```python
from build123d import *

# Parameters (mm, degrees)
SZKIC2_W                    = 62
SZKIC2_H                    = 5
SZKIC3_R                    = 1.45
DODANIE_WYCI_GNI_CIE1_DEPTH = 5
SFAZOWANIE1_SIZE            = 4
ZAOKR_GLENIE1_R             = 2
SFAZOWANIE2_SIZE            = 0.5


with BuildPart() as part:
    # Szkic2 → Obrót1 (revolve)
    with BuildSketch(Plane.XY):
        Polygon((15, 15), (15, 5), (25, 5), (25, 25), (8.15, 25), (8.15, 15), align=None)
        with Locations((46, 2.5)):
            Rectangle(SZKIC2_W, SZKIC2_H)
    revolve(axis=Axis((0, 0, 0), (0, 1, 0)))

    # Szkic3 → Dodanie-wyciągnięcie1 (add)
    with BuildSketch(Plane(origin=(0, 5, 0), x_dir=(1, 0, 0), z_dir=(0, 1, 0))):
        with BuildLine():
            Line((-4, 76.5), (-4, 79))
            ThreePointArc((-4, 79), (0, 83), (4, 79))
            Line((4, 79), (4, 76.5))
            ThreePointArc((4, 76.5), (0, 72.5), (-4, 76.5))
        make_face()
        with Locations((0, 79)):
            Circle(SZKIC3_R, mode=Mode.SUBTRACT)
        with BuildLine():
            Line((76.5, 4), (79, 4))
            ThreePointArc((79, 4), (83, 0), (79, -4))
            Line((79, -4), (76.5, -4))
            ThreePointArc((76.5, -4), (72.5, 0), (76.5, 4))
        make_face()
        with Locations((79, 0)):
            Circle(SZKIC3_R, mode=Mode.SUBTRACT)
        with BuildLine():
            Line((4, -76.5), (4, -79))
            ThreePointArc((4, -79), (0, -83), (-4, -79))
            Line((-4, -79), (-4, -76.5))
            ThreePointArc((-4, -76.5), (0, -72.5), (4, -76.5))
        make_face()
        with Locations((0, -79)):
            Circle(SZKIC3_R, mode=Mode.SUBTRACT)
        with BuildLine():
            Line((-76.5, -4), (-79, -4))
            ThreePointArc((-79, -4), (-83, 0), (-79, 4))
            Line((-79, 4), (-76.5, 4))
            ThreePointArc((-76.5, 4), (-72.5, 0), (-76.5, -4))
        make_face()
        with Locations((-79, 0)):
            Circle(SZKIC3_R, mode=Mode.SUBTRACT)
    extrude(amount=-DODANIE_WYCI_GNI_CIE1_DEPTH)

    # Sfazowanie1
    sfazowanie1_edges = [part.edges().sort_by_distance(p)[0] for p in [
        (-25, 25, 0),
        (-25, 5, 0),
    ]]
    chamfer(sfazowanie1_edges, length=SFAZOWANIE1_SIZE)

    # Zaokrąglenie1
    zaokr_glenie1_edges = [part.edges().sort_by_distance(p)[0] for p in [
        (-76.896033708, 2.5, -4),
        (-76.896033708, 2.5, 4),
        (-4, 2.5, 76.896033708),
        (4, 2.5, 76.896033708),
        (76.896033708, 2.5, 4),
        (76.896033708, 2.5, -4),
        (4, 2.5, -76.896033708),
        (-4, 2.5, -76.896033708),
    ]]
    fillet(zaokr_glenie1_edges, radius=ZAOKR_GLENIE1_R)

    # Sfazowanie2
    sfazowanie2_edges = [part.edges().sort_by_distance(p)[0] for p in [
        (4, 5, -78.885911187),
        (4, 0, -78.885911187),
        (-4, 5, -78.885911187),
        (-4, 0, -78.885911187),
        (77.41237349, 5, 4.53306485),
        (77.41237349, 0, 4.53306485),
        (77.41237349, 5, -4.53306485),
        (77.41237349, 0, -4.53306485),
        (4.53306485, 5, 77.41237349),
        (4.53306485, 0, 77.41237349),
        (-4.53306485, 5, 77.41237349),
        (-4.53306485, 0, 77.41237349),
        (-77.41237349, 5, 4.53306485),
        (-77.41237349, 0, 4.53306485),
        (-77.41237349, 5, -4.53306485),
        (-77.41237349, 0, -4.53306485),
        (4.53306485, 5, -77.41237349),
        (4.53306485, 0, -77.41237349),
        (-4.53306485, 5, -77.41237349),
        (-4.53306485, 0, -77.41237349),
        (-83, 0, 0),
        (-80.45, 0, 0),
        (-83, 5, 0),
        (0, 0, 83),
        (-1.45, 0, 79),
        (0, 5, 83),
        (83, 0, 0),
        (77.55, 0, 0),
        (83, 5, 0),
        (0, 0, -83),
        (-1.45, 0, -79),
        (0, 5, -83),
        (-15, 0, 0),
        (54.447222151, 5, 54.447222151),
        (54.447222151, 0, 54.447222151),
        (78.885911187, 5, 4),
        (78.885911187, 0, 4),
        (78.885911187, 5, -4),
        (78.885911187, 0, -4),
        (54.447222151, 5, -54.447222151),
        (54.447222151, 0, -54.447222151),
        (4, 5, 78.885911187),
        (4, 0, 78.885911187),
        (-54.447222151, 5, 54.447222151),
        (-54.447222151, 0, 54.447222151),
        (-4, 5, 78.885911187),
        (-4, 0, 78.885911187),
        (-78.885911187, 5, 4),
        (-78.885911187, 0, 4),
        (-54.447222151, 5, -54.447222151),
        (-54.447222151, 0, -54.447222151),
        (-78.885911187, 5, -4),
        (-78.885911187, 0, -4),
    ]]
    chamfer(sfazowanie2_edges, length=SFAZOWANIE2_SIZE)


solid = part.part
```
Input: part model. Units: mm. Frame: model coordinates. A direction names the side the tool comes from. Give positions to 0.01 mm unless a question says otherwise; leave off trailing zeros. Write each question's results on one line, items separated by ' | '. Start each with the question number.
Item 1: Set-up query: faces 1 (the cylindrical face through (23.846, 15.084, -7.509)), 2 (the conical face through (-0.08, 0.135, -82.635)). Return all of +Z, -Z, +X, -X, +Y, -Y with unobstructed straight access to the full face (end or side cutting, diameter ignored); none if empty.
Item 2: Line query: line 1 (X direction, y = 3.05, z = 0); line 2 (Z direction, x = 79, y = 3.95). Output: solid intervals per line, ascending.
Item 3: Contact query for flat-ended pins moving along their axis: P1, Ø14.5, axis at x = 0, z = 0, coming from the +Y side; P2, Ø12, axis at x = 65, y = 7, coming from the +Z side; P3, Ø4, axis at x = 29, z = 63.5, coming from the -Y side; P4, Ø3, axis at x = -65, y = 3.5, coming from the -Z side. Output: stop coordinate, or through.
Item 4: Mould query, pull axis X, two halves, no side actions, for faces 3 (the conical face through (82.635, 0.135, -0.08)), 4 (the conical face through (0.08, 4.86, 82.64)), 5 (the cylindrical face through (-14.985, 7.648, -0.66)). Classes: pulls with the +X half, pulls with the -X half, needs draft (parallel to the pull), parting line crosses it, or undercut.
Established:
1) face 1: +Y | face 2: -Z, -Y
2) line 1: -83 to -80.45, -77.55 to -15, 15 to 77.55, 80.45 to 83 | line 2: -4 to -1.45, 1.45 to 4
3) P1: through | P2: z = 48.82 | P3: y = 0 | P4: z = -43.55
4) face 3: pulls with the +X half | face 4: parting line crosses it | face 5: undercut
